The drawing under review shows one solid part. Ordinate dimensions are in mm from its lowest x, y, z. A direction names the side the tool comes from. Coordinates: 2 decimals unless noted, no trailing zeros. Order: outer loops, then holes, each group sorted by start corner. A loop starts at its lowest first (then second) coordinate and runs counter-clockwise, first axis right, second up. Notation, with made-up numbers: (33.25, -20) - (64.25, -20) arc R4 cw to (64.25, -15) - close; hole circle Ø3 at (20.25, 5.5). An arc over 180 degrees is marked (long way). Write each question's results on one line, items separated by ' | '. Start each with the question number.
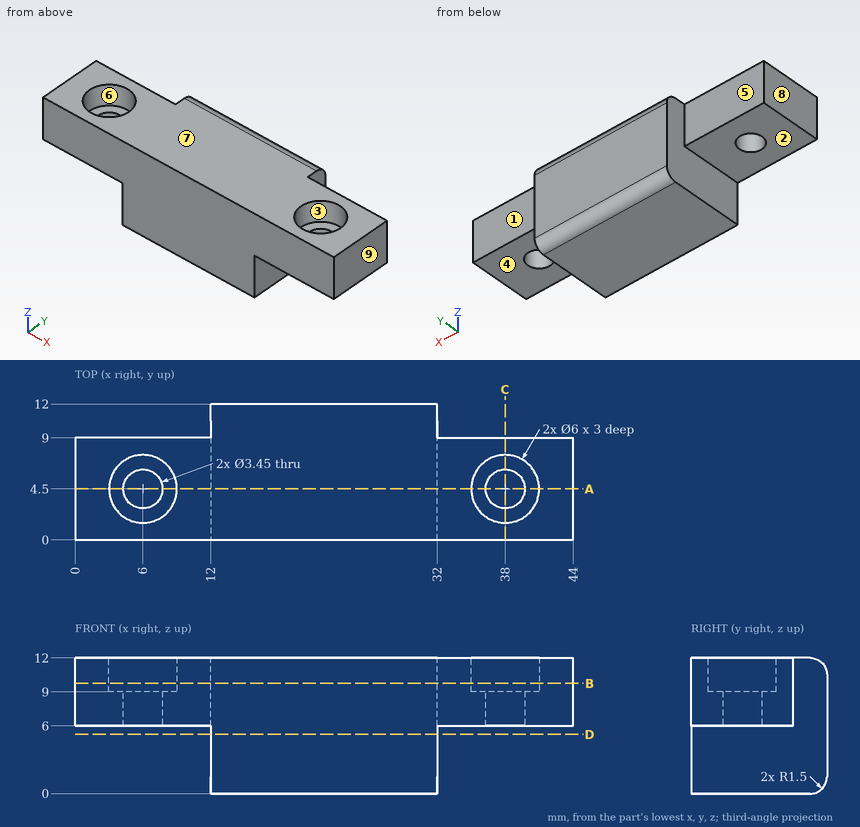
(1) Tool access review of the marked faces 1, 2, 3, 4 and 5: name each direction out of +Z, -Z, +X, -X, +Y, -Y from which nothing blocks a thin tool from reaching the whole face with its end or side.
(2) Take a section at C-C (x = 38). State the section outline as (y, z) points (3 decimals).
(3) Take a section at B-B (z = 9.75). State the section outline as (x, y) points, plus the area to 3 significant figures.
(4) Take a section at D-D (z = 5.25). State the section outline as (x, y) points, plus the area to 3 significant figures.
(5) Mouldability with a two-part tool opening along X and no side actions: class the marked faces 6, 7, 8 and 9 as +X half, -X half, draft (parallel to the pull), parting line (faces both ways), or undercut.
(6) To check wall thickness, follow line 1 along Y through (x, z) = (6, 7) (3 decimals); line 2 along Y through (x, z) = (38, 9.85); line 3 along X through (y, z) = (2.75, 10.5). State the ranges of each line that lie inside material, in increasing order. Write a range as [from, to].
(7) Take a section at A-A (y = 4.5). State the section outline as (x, z) points (3 decimals), plus the area to 3 significant figures.
(8) Clearance check with flat-ended pins moving along their axes: pin 1 (4 mm diameter, centred on x = 6.5, y = 3.5, fed in from -Z); pin 2 (1.8 mm diameter, centred on x = 36.5, z = 8.5, fed in from +Y); pin 3 (1.5 mm diameter, centred on y = 4, z = 4.5, fed in from -X). State where each tip first meets the part, or that it passes through.
Worked out:
1) face 1: +Z, -Z, +X, +Y | face 2: -Z, -X, +Y, -Y | face 3: +Z | face 4: -Z, +X, +Y, -Y | face 5: +Z, -Z, -X, +Y
2) outline: (0, 6) - (2.775, 6) - (2.775, 9) - (1.5, 9) - (1.5, 12) - (0, 12) - close; (6.225, 6) - (9, 6) - (9, 12) - (7.5, 12) - (7.5, 9) - (6.225, 9) - close
3) outline: (0, 0) - (44, 0) - (44, 9) - (32, 9) - (32, 12) - (12, 12) - (12, 9) - (0, 9) - close; hole circle Ø6 at (6, 4.5); hole circle Ø6 at (38, 4.5) | area: 399 mm^2
4) outline: (12, 0) - (32, 0) - (32, 12) - (12, 12) - close | area: 240 mm^2
5) face 6: undercut | face 7: draft | face 8: -X half | face 9: +X half
6) line 1: [0, 2.775], [6.225, 9] | line 2: [0, 1.5], [7.5, 9] | line 3: [0, 3.56], [8.44, 35.56], [40.44, 44]
7) outline: (0, 6) - (4.275, 6) - (4.275, 9) - (3, 9) - (3, 12) - (0, 12) - close; (7.725, 6) - (12, 6) - (12, 0) - (32, 0) - (32, 6) - (36.275, 6) - (36.275, 9) - (35, 9) - (35, 12) - (9, 12) - (9, 9) - (7.725, 9) - close; (39.725, 6) - (44, 6) - (44, 12) - (41, 12) - (41, 9) - (39.725, 9) - close | area: 327 mm^2
8) pin 1: z = 6 | pin 2: y = 9 | pin 3: x = 12
